Design review of the part built by this model. Coordinates are the model's own, in mm. A direction names the side the tool comes from. Give positions to 0.01 mm unless a question says otherwise; leave off trailing zeros. Loops run counter-clockwise (first coordinate to the right, second up) from the corner with the lowest first, then second, coordinate; pieces in that order, holes last. Notation, with made-up numbers: (-25.5, 68) - (21.5, 68) arc R29 ccw to (21.5, 102) - close; hole circle Ø7 at (-40, -14.75). An arc over 180 degrees is marked (long way). Write each question's results on one line, items separated by ' | '.
```python
from build123d import *

# Parameters (mm, degrees)
F0_R     = 1.5
F1_DEPTH = 14
F2_DEPTH = 14
F3_R     = 1.5
F4_DEPTH = 3
F5_R     = 1.5
F6_DEPTH = 5


with BuildPart() as f1:
    # F0 (on Top) → F1 (new body, symmetric)
    with BuildSketch(Plane.XY):
        Polygon((3.590729, -0.580228), (2.297857, 2.819549), (-1.292872, 3.399777), (-3.590729, 0.580228), (-2.297857, -2.819549), (1.292872, -3.399777), align=None)
        Circle(F0_R, mode=Mode.SUBTRACT)
    extrude(amount=F1_DEPTH, both=True)

    # F0 (on Top) → F2 (join, symmetric)
    with BuildSketch(Plane.XY):
        Circle(F0_R)
    extrude(amount=F2_DEPTH, both=True)

    # F3 (on face) → F4 (join)
    with BuildSketch(Plane(origin=(0, 0, -14), x_dir=(1, 0, 0), z_dir=(0, 0, -1))):
        Circle(F3_R)
    extrude(amount=F4_DEPTH)

    # F5 (on face) → F6 (join)
    with BuildSketch(Plane.XY.offset(14)):
        Circle(F5_R)
    extrude(amount=F6_DEPTH)


solid = f1.part
```
Item 1: We need section D-D on y = 2.5. Give the boundary of the cut face in (x, z), then the cut area to 3 significant figures.
Output values:
outline: (-2.03, -14) - (2.42, -14) - (2.42, 14) - (-2.03, 14) - close | area: 124 mm²
Item 2: We need section C-C on y = 0. Give the boundary of the cut face in (x, z), then the cut area to 3 significant figures.
Output values:
outline: (-3.37, -14) - (-1.5, -14) - (-1.5, -17) - (1.5, -17) - (1.5, -14) - (3.37, -14) - (3.37, 14) - (1.5, 14) - (1.5, 19) - (-1.5, 19) - (-1.5, 14) - (-3.37, 14) - close | area: 213 mm²
Item 3: Wall thickness on probe 1 along Z at (x, y) = (2, -2.25); probe 2 along X at (y, z) = (0, 12.5); probe 3 along Y at (x, z) = (2.25, 2.5): over which ranges is each line inside the solid? List them lowest first.
Output values:
probe 1: z = -14 to 14 | probe 2: x = -3.37 to 3.37 | probe 3: y = -2.23 to 2.83
Item 4: Tool access review of faces 1 (the face through (2.95, 1.1, 0.2)), 2 (the face through (0, 2, 14)), 3 (the face through (0, 2, -14)): name each direction out of +Z, -Z, +X, -X, +Y, -Y from which nothing blocks a thin tool from reaching the whole face with its end or side.
Output values:
face 1: +Z, -Z, +X, +Y | face 2: +Z | face 3: -Z
Item 5: We need section A-A on x = -0.25. Give the boundary of the cut face in (y, z).
Output values:
outline: (-3.15, -14) - (-1.48, -14) - (-1.48, -17) - (1.48, -17) - (1.48, -14) - (3.23, -14) - (3.23, 14) - (1.48, 14) - (1.48, 19) - (-1.48, 19) - (-1.48, 14) - (-3.15, 14) - close
Item 6: Clearance check with flat-ended pins moving along their axes: P1, Ø2, axis at y = -2, z = -5, coming from the -X side; P2, Ø3, axis at x = -2, y = -2.5, coming from the +Z side; P3, Ø1, axis at x = -1.5, z = 5, coming from the -Y side. State where each tip first meets the part, or that it passes through.
Output values:
P1: stops at x = -2.99 | P2: stops at z = 14 | P3: stops at y = -3.03
Item 7: We need section B-B on z = -15. Give the boundary of the cut face in (x, y).
Output values:
outline: circle Ø3 at (0, 0)
